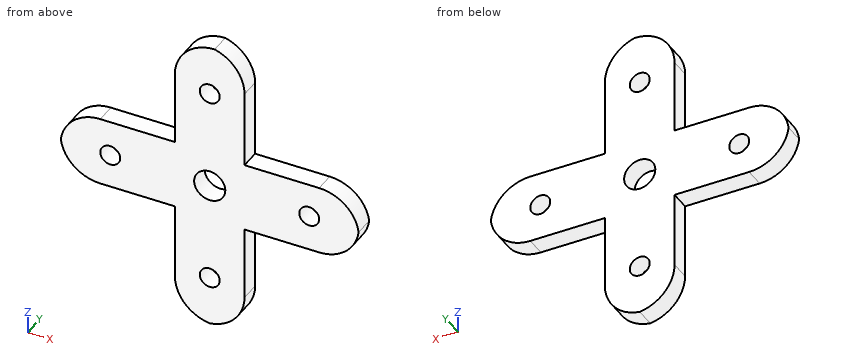
```python
from build123d import *

# Parameters (mm, degrees)
BOSS_EXTRUDE1_DEPTH = 2.54
FILLET1_R           = 5.08
FILLET2_R           = 5.08
SKETCH2_R           = 1.989538673
SKETCH2_R_2         = 1.27
CUT_EXTRUDE1_DEPTH  = 2.54


with BuildPart() as part:
    # Sketch1 → Boss-Extrude1 (new body)
    with BuildSketch(Plane(origin=(0, 0, 0), x_dir=(1, 0, 0), z_dir=(0, 1, 0))):
        Polygon((-4.200769231, 17.994923077), (-4.200769231, 3.262923077), (-18.805769231, 3.262923077), (-18.805769231, -5.627076923), (-4.200769231, -5.627076923), (-4.200769231, -20.105076923), (4.689230769, -20.105076923), (4.689230769, -5.373076923), (19.294230769, -5.373076923), (19.294230769, 3.516923077), (4.689230769, 3.516923077), (4.689230769, 17.994923077), align=None)
    extrude(amount=BOSS_EXTRUDE1_DEPTH)

    # Fillet1
    fillet1_edges = [part.edges().sort_by_distance(p)[0] for p in [
        (-4.200769231, 1.27, 20.105076923),
    ]]
    fillet(fillet1_edges, radius=FILLET1_R)

    # Fillet2
    # the kernel refuses this fillet: 5.08 mm, written as the material it takes off along each edge
    with BuildSketch(Plane(origin=(-4.200769231, -12.7, -17.994923077), x_dir=(0, 0, 1), z_dir=(0, 1, 0)), Plane(origin=(-18.805769231, -12.7, -3.262923077), x_dir=(0, 0, 1), z_dir=(0, 1, 0)), Plane(origin=(-18.805769231, -12.7, 5.627076923), x_dir=(1, 0, 0), z_dir=(0, 1, 0)), Plane(origin=(4.689230769, -12.7, -17.994923077), x_dir=(-1, 0, 0), z_dir=(0, 1, 0))) as fillet2_piece_1:
        with BuildLine():
            CenterArc((FILLET2_R, FILLET2_R), FILLET2_R, 180, 90)
            Line((0, FILLET2_R), (-FILLET2_R * 0.02, FILLET2_R))
            Line((-FILLET2_R * 0.02, FILLET2_R), (-FILLET2_R * 0.02, -FILLET2_R * 0.02))
            Line((-FILLET2_R * 0.02, -FILLET2_R * 0.02), (FILLET2_R, -FILLET2_R * 0.02))
            Line((FILLET2_R, -FILLET2_R * 0.02), (FILLET2_R, 0))
        make_face()
    extrude(amount=27.94, mode=Mode.SUBTRACT)
    with BuildSketch(Plane(origin=(19.294230769, -12.7, -3.516923077), x_dir=(0, 0, 1), z_dir=(0, 1, 0)), Plane(origin=(19.294230769, -12.7, 5.373076923), x_dir=(-1, 0, 0), z_dir=(0, 1, 0))) as fillet2_piece_2:
        with BuildLine():
            CenterArc((FILLET2_R, -FILLET2_R), FILLET2_R, 90, 90)
            Line((0, -FILLET2_R), (-FILLET2_R * 0.02, -FILLET2_R))
            Line((-FILLET2_R * 0.02, -FILLET2_R), (-FILLET2_R * 0.02, FILLET2_R * 0.02))
            Line((-FILLET2_R * 0.02, FILLET2_R * 0.02), (FILLET2_R, FILLET2_R * 0.02))
            Line((FILLET2_R, FILLET2_R * 0.02), (FILLET2_R, 0))
        make_face()
    extrude(amount=27.94, mode=Mode.SUBTRACT)
    with BuildSketch(Plane(origin=(4.689230769, -12.296722124, 20.105076923), x_dir=(-1, 0, 0), z_dir=(0, 1, 0))) as fillet2_piece_3:
        with BuildLine():
            CenterArc((5.08, -4.91868885), FILLET2_R, 104.477512186, 75.522487814)
            Line((0, -4.91868885), (-0.1016, -4.91868885))
            Line((-0.1016, -4.91868885), (-0.1016, 0))
            Line((-0.1016, 0), (0, 0.1016))
            ThreePointArc((0, 0.1016), (1.905, 0.1016), (3.7846, 0.098373777))
            Line((3.7846, 0.098373777), (3.81, 0))
        make_face()
    extrude(amount=27.133444248, mode=Mode.SUBTRACT)

    # Sketch2 → Cut-Extrude1 (cut)
    with BuildSketch(Plane(origin=(0, 2.54, 0), x_dir=(1, 0, 0), z_dir=(0, 1, 0))):
        with Locations(Location((0.244230769, -1.055076923, 0), (0, 0, 270))):
            Circle(SKETCH2_R)
        with Locations(Location((0.244230769, 11.644923077, 0), (0, 0, 270))):
            Circle(SKETCH2_R_2)
        with Locations(Location((0.244230769, -13.755076923, 0), (0, 0, 270))):
            Circle(SKETCH2_R_2)
        with Locations(Location((-12.455769231, -1.055076923, 0), (0, 0, 270))):
            Circle(SKETCH2_R_2)
        with Locations(Location((12.944230769, -1.055076923, 0), (0, 0, 270))):
            Circle(SKETCH2_R_2)
    extrude(amount=-CUT_EXTRUDE1_DEPTH, mode=Mode.SUBTRACT)


solid = part.part
```
Work out the finished part from the listing and answer in its coordinate system (mm). Coordinates: 2 decimals unless noted, no trailing zeros. Loops run counter-clockwise (first coordinate to the right, second up) from the corner with the lowest first, then second, coordinate; pieces in that order, holes last. Notation, with made-up numbers: (60.5, 62) -> (78.5, 62) arc R11 ccw to (78.5, 77) -> close; hole circle Ø1 at (15.5, 55). An arc over 180 degrees is marked (long way). Answer as CSV lines item,"result".
Q1. The part is cut by section B-B on x = 7. Write down the section's boundary in (y, z), and give its area (3 significant figures).
Findings:
outline,"(0, -3.52) -> (2.54, -3.52) -> (2.54, 5.37) -> (0, 5.37) -> close"
area,"22.6 mm²"
Q2. Find the intervals of material crossed by probe 1 along X at (y, z) = (0.35, 2); probe 2 along Z at (x, y) = (-5, 1.4); probe 3 along X at (y, z) = (0.25, 11), in increasing order.
Findings:
probe 1,"x = -18.59 to -13.3, -11.61 to -1.51, 2 to 12.1, 13.79 to 19"
probe 2,"z = -3.26 to 5.63"
probe 3,"x = -4.2 to 4.69"
Q3. The part is cut by section C-C on z = 10. Write down the section's boundary in (x, y).
Findings:
outline,"(-4.2, 0) -> (4.69, 0) -> (4.69, 2.54) -> (-4.2, 2.54) -> close"
Q4. The part is cut by section A-A on y = 0.45. Write down the section's boundary in (x, z), and give its area (3 significant figures).
Findings:
outline,"(-18.77, 1.18) arc R5.08 ccw to (-13.73, -3.26) -> (-4.2, -3.26) -> (-4.2, -12.91) arc R5.08 ccw to (0.24, -17.96) arc R5.08 ccw to (4.69, -12.91) -> (4.69, -3.52) -> (14.21, -3.52) arc R5.08 ccw to (19.25, 0.93) arc R5.08 ccw to (14.21, 5.37) -> (4.69, 5.37) -> (4.69, 15.19) arc R5.08 ccw to (0.88, 20.11) arc R5.08 ccw to (-4.2, 15.03) -> (-4.2, 5.63) -> (-13.73, 5.63) arc R5.08 ccw to start; hole circle Ø2.54 at (-12.46, 1.06); hole circle Ø3.98 at (0.24, 1.06); hole circle Ø2.54 at (0.24, -11.64); hole circle Ø2.54 at (0.24, 13.76); hole circle Ø2.54 at (12.94, 1.06)"
area,"522 mm²"
Q5. Each of these flat-tipped pins is pushed along its axis until it touches: pin 1 (1.3 mm diameter, centred on y = 1, z = 8.5, fed in from +X); pin 2 (1.3 mm diameter, centred on x = 8.5, y = 1.5, fed in from -Z); pin 3 (2 mm diameter, centred on x = 0.24, z = -11.64, fed in from -Y); pin 4 (1 mm diameter, centred on y = 0.5, z = 2, fed in from +X). Where does it stop, or does it pass through?
Findings:
pin 1,"stops at x = 4.69"
pin 2,"stops at z = -3.52"
pin 3,"passes through"
pin 4,"stops at x = 19.15"
